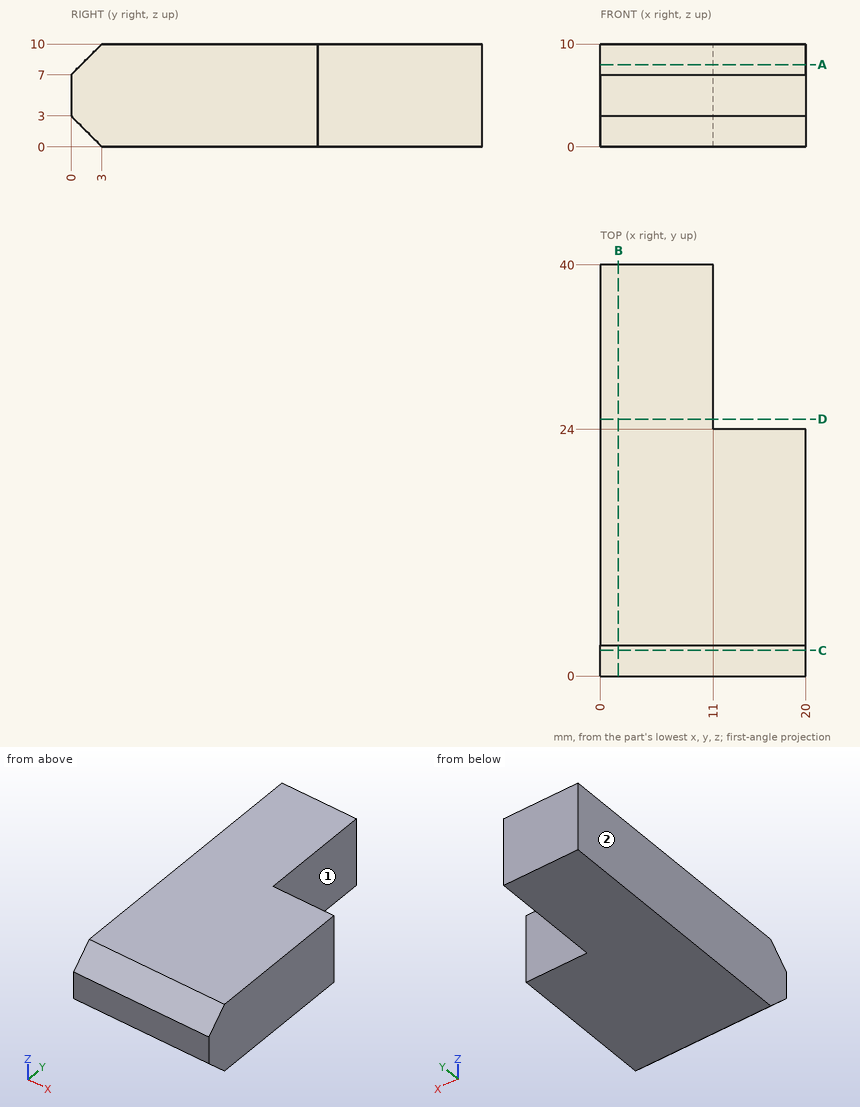
Print and shaded views of the part. All mm, measured from the part's lowest x, y and z. A direction names the side the tool comes from. Round coordinates to 2 decimals unless told otherwise and drop trailing zeros. Write each loop counter-clockwise with the first axis right and the second up, starting at its lowest first coordinate (ties: lowest second). Pieces come first, ordered by that corner, then holes.
(1) Slice it at C-C, the plane y = 2.5. Write the cut outline in (x, z), and give its area (3 significant figures).
(2) 3-axis set-ups, long thin cutter, end or side, ignore diameter. For the marked faces 1 and 2: which of +Z, -Z, +X, -X, +Y, -Y reach the whole face in a straight line?
(3) Slice it at D-D, the plane y = 25. Write the cut outline in (x, z), and give its area (3 significant figures).
(4) Probe line 1 along Y through (x, z) = (17, 3.75); line 2 along X through (y, z) = (36, 7); line 3 along Z through (x, y) = (2.75, 2.5). List the from-to ranges inside material, lowest first.
(5) Slice it at A-A, the plane z = 8. Write the cut outline in (x, y), and give its area (3 significant figures).
(6) Drop a flat-ended pin along its axis: P1, Ø5, axis at y = 33.5, z = 6, coming from the +X side. Give the stop position or say it passes through.
(7) Slice it at B-B, the plane x = 1.75. Write the cut outline in (y, z).
From the geometry:
1. outline: (0, 0.5) - (20, 0.5) - (20, 9.5) - (0, 9.5) - close
1. area: 180 mm2
2. face 1: +Z, -Z, +X, +Y
2. face 2: +Z, -Z, -X, +Y, -Y
3. outline: (0, 0) - (11, 0) - (11, 10) - (0, 10) - close
3. area: 110 mm2
4. line 1: y = 0 to 24
4. line 2: x = 0 to 11
4. line 3: z = 0.5 to 9.5
5. outline: (0, 1) - (20, 1) - (20, 24) - (11, 24) - (11, 40) - (0, 40) - close
5. area: 636 mm2
6. P1: stops at x = 11
7. outline: (0, 3) - (3, 0) - (40, 0) - (40, 10) - (3, 10) - (0, 7) - close
